```python
from build123d import *

# Parameters (mm, degrees)
F1_DEPTH = 2
F2_DEPTH = 19
F3_R     = 3.678544
F3_R_2   = 2.75
F3_R_3   = 4.215462
F3_R_4   = 4.179516
F3_R_5   = 4.278838
F4_DEPTH = 5
F5_W     = 2
F5_H     = 15.1
F5_H_2   = 15.9
F5_W_2   = 9
F5_H_3   = 2
F5_W_3   = 17
F5_W_4   = 8
F6_DEPTH = 12
F7_W     = 15.6
F7_H     = 4
F8_DEPTH = 2


with BuildPart() as f1:
    # F0 (on Top) → F1 (new body)
    with BuildSketch(Plane.XY):
        with BuildLine():
            Line((88.5, 0), (2.5, 0))
            ThreePointArc((2.5, 0), (0.732233, -0.732233), (0, -2.5))
            Line((0, -2.5), (0, -59.5))
            ThreePointArc((0, -59.5), (0.732233, -61.267767), (2.5, -62))
            Line((2.5, -62), (88.5, -62))
            ThreePointArc((88.5, -62), (90.267767, -61.267767), (91, -59.5))
            Line((91, -59.5), (91, -2.5))
            ThreePointArc((91, -2.5), (90.267767, -0.732233), (88.5, 0))
        make_face()
        with BuildLine():
            ThreePointArc((2, -2.5), (2.146447, -2.146447), (2.5, -2))
            Line((2.5, -2), (88.5, -2))
            ThreePointArc((88.5, -2), (88.853553, -2.146447), (89, -2.5))
            Line((89, -2.5), (89, -59.5))
            ThreePointArc((89, -59.5), (88.853553, -59.853553), (88.5, -60))
            Line((88.5, -60), (2.5, -60))
            ThreePointArc((2.5, -60), (2.146447, -59.853553), (2, -59.5))
            Line((2, -59.5), (2, -2.5))
        make_face(mode=Mode.SUBTRACT)
        with BuildLine():
            Line((88.5, -2), (2.5, -2))
            ThreePointArc((2.5, -2), (2.146447, -2.146447), (2, -2.5))
            Line((2, -2.5), (2, -59.5))
            ThreePointArc((2, -59.5), (2.146447, -59.853553), (2.5, -60))
            Line((2.5, -60), (88.5, -60))
            ThreePointArc((88.5, -60), (88.853553, -59.853553), (89, -59.5))
            Line((89, -59.5), (89, -2.5))
            ThreePointArc((89, -2.5), (88.853553, -2.146447), (88.5, -2))
        make_face()
    extrude(amount=F1_DEPTH)

    # F0 (on Top) → F2 (join)
    with BuildSketch(Plane.XY):
        with BuildLine():
            Line((88.5, 0), (2.5, 0))
            ThreePointArc((2.5, 0), (0.732233, -0.732233), (0, -2.5))
            Line((0, -2.5), (0, -59.5))
            ThreePointArc((0, -59.5), (0.732233, -61.267767), (2.5, -62))
            Line((2.5, -62), (88.5, -62))
            ThreePointArc((88.5, -62), (90.267767, -61.267767), (91, -59.5))
            Line((91, -59.5), (91, -2.5))
            ThreePointArc((91, -2.5), (90.267767, -0.732233), (88.5, 0))
        make_face()
        with BuildLine():
            ThreePointArc((2, -2.5), (2.146447, -2.146447), (2.5, -2))
            Line((2.5, -2), (88.5, -2))
            ThreePointArc((88.5, -2), (88.853553, -2.146447), (89, -2.5))
            Line((89, -2.5), (89, -59.5))
            ThreePointArc((89, -59.5), (88.853553, -59.853553), (88.5, -60))
            Line((88.5, -60), (2.5, -60))
            ThreePointArc((2.5, -60), (2.146447, -59.853553), (2, -59.5))
            Line((2, -59.5), (2, -2.5))
        make_face(mode=Mode.SUBTRACT)
    extrude(amount=F2_DEPTH)

    # F3 (on face) → F4 (join)
    with BuildSketch(Plane.XY.offset(2)):
        with Locations((6.5, -6.5)):
            Circle(F3_R)
        with Locations((6.5, -6.5)):
            Circle(F3_R_2, mode=Mode.SUBTRACT)
        with Locations((64.5, -6.5)):
            Circle(F3_R_3)
        with Locations((64.5, -6.5)):
            Circle(F3_R_2, mode=Mode.SUBTRACT)
        with Locations((6.5, -55.5)):
            Circle(F3_R_4)
        with Locations((6.5, -55.5)):
            Circle(F3_R_2, mode=Mode.SUBTRACT)
        with Locations((64.5, -55.5)):
            Circle(F3_R_5)
        with Locations((64.5, -55.5)):
            Circle(F3_R_2, mode=Mode.SUBTRACT)
    extrude(amount=F4_DEPTH)

    # F5 (on face) → F6 (cut)
    with BuildSketch(Plane.XY.offset(19)):
        with Locations((90, -12.05)):
            Rectangle(F5_W, F5_H)
        with Locations((90, -31.05)):
            Rectangle(F5_W, F5_H)
        with Locations((90, -48.75)):
            Rectangle(F5_W, F5_H_2)
        with Locations((13.55, -61)):
            Rectangle(F5_W_2, F5_H_3)
        with Locations((35, -61)):
            Rectangle(F5_W_3, F5_H_3)
        with Locations((57.25, -61)):
            Rectangle(F5_W_4, F5_H_3)
    extrude(amount=-F6_DEPTH, mode=Mode.SUBTRACT)

    # F7 (on face) → F8 (cut)
    with BuildSketch(Plane(origin=(0, 0, 0), x_dir=(0, -1, 0), z_dir=(-1, 0, 0))):
        with Locations((30.3, 6)):
            Rectangle(F7_W, F7_H)
    extrude(amount=-F8_DEPTH, mode=Mode.SUBTRACT)


solid = f1.part
```
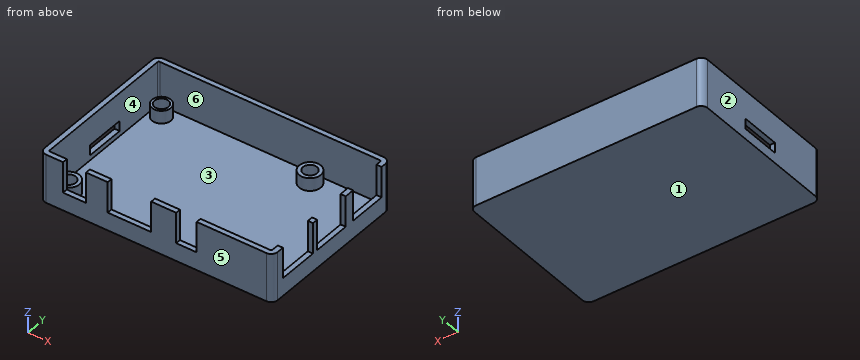
The model under review builds one solid part; all positions refer to its coordinate system, in mm. Face numbers are marked on the shaded views. A direction names the side the tool comes from. Give positions to 0.01 mm unless a question says otherwise; leave off trailing zeros. Write each loop counter-clockwise with the first axis right and the second up, starting at its lowest first coordinate (ties: lowest second). Pieces come first, ordered by that corner, then holes. Notation, with made-up numbers: (85.5, 84) - (107.5, 84) arc R23 ccw to (107.5, 107) - close; hole circle Ø8 at (-19.5, 55). An arc over 180 degrees is marked (long way). Answer in a Markdown table with one row per item. Add a question column.
1. Insertion check: P1, Ø5, axis at x = 18.5, y = -26.5, coming from the +Z side; P2, Ø6, axis at x = 7.5, y = -55, coming from the +Z side; P3, Ø2, axis at y = -29.5, z = 10.5, coming from the +X side. Each pin has a flat end and moves straight along its axis. Give the tip position at first contact, or say it passes through.
2. We need section B-B on y = -6.5. Write out the cut boundary in (x, z).
3. Tool access review of the marked faces 5 and 6: name each direction out of +Z, -Z, +X, -X, +Y, -Y from which nothing blocks a thin tool from reaching the whole face with its end or side.
4. We need section A-A on z = 5.25. State how many separate pieces and enclosed holes the cut face has, then the cut area to 3 significant figures.
5. We need section C-C on x = 6.5. Write out the cut boundary in (y, z).
6. Draft analysis for pull direction X (two halves, no side actions). For the marked faces 1, 2, 3 and 4, state which applies: +X half, -X half, draft (parallel to the pull), parting line (faces both ways), or undercut.
7. Wall thickness on line 1 along Y through (x, z) = (6.5, 5.15); line 2 along Y through (x, z) = (64.5, 3.65); line 3 along Y through (x, z) = (28, 4): over which ranges is each line inside the solid? List them lowest first. Write a range as [from, to].
Ans:
| question | item | result |
|---|---|---|
| 1 | P1 | stops at z = 2 |
| 1 | P2 | stops at z = 7 |
| 1 | P3 | stops at x = 2 |
| 2 | outline | (0, 0) - (91, 0) - (91, 7) - (89, 7) - (89, 2) - (68.72, 2) - (68.72, 7) - (67.25, 7) - (67.25, 2) - (61.75, 2) - (61.75, 7) - (60.28, 7) - (60.28, 2) - (10.18, 2) - (10.18, 7) - (9.25, 7) - (9.25, 2) - (3.75, 2) - (3.75, 7) - (2.82, 7) - (2.82, 2) - (2, 2) - (2, 19) - (0, 19) - close |
| 3 | face 5 | +Z, -Z, +X, -X, -Y |
| 3 | face 6 | +Z |
| 4 | separate pieces | 5 |
| 4 | enclosed holes | 4 |
| 4 | area | 675 mm^2 |
| 5 | outline | (-62, 0) - (0, 0) - (0, 19) - (-2, 19) - (-2, 2) - (-2.82, 2) - (-2.82, 7) - (-3.75, 7) - (-3.75, 2) - (-9.25, 2) - (-9.25, 7) - (-10.18, 7) - (-10.18, 2) - (-51.32, 2) - (-51.32, 7) - (-52.75, 7) - (-52.75, 2) - (-58.25, 2) - (-58.25, 7) - (-59.68, 7) - (-59.68, 2) - (-60, 2) - (-60, 19) - (-62, 19) - close |
| 6 | face 1 | draft |
| 6 | face 2 | -X half |
| 6 | face 3 | undercut |
| 6 | face 4 | undercut |
| 7 | line 1 | y = [-62, -60], [-59.68, -58.25], [-52.75, -51.32], [-10.18, -9.25], [-3.75, -2.82], [-2, 0] |
| 7 | line 2 | y = [-62, -60], [-59.78, -58.25], [-52.75, -51.22], [-10.72, -9.25], [-3.75, -2.28], [-2, 0] |
| 7 | line 3 | y = [-62, -60], [-2, 0] |
